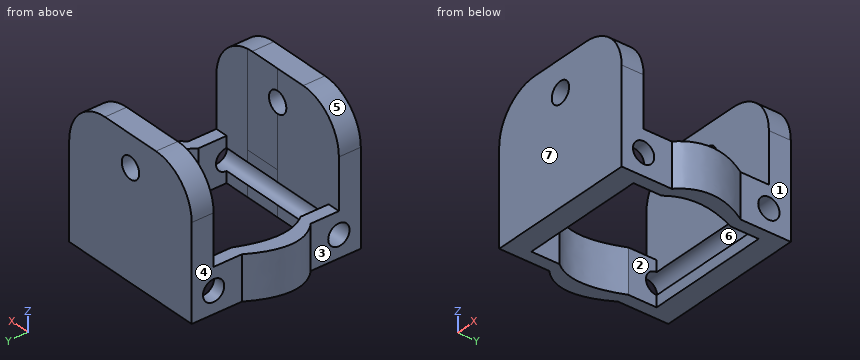
```python
from build123d import *

# Parameters (mm, degrees)
SKETCH1_W               = 24
SKETCH1_H               = 3.5
BOSS_EXTRUDE1_DEPTH     = 7
BOSS_EXTRUDE2_START     = 7
BOSS_EXTRUDE2_OUTLINE_W = 24
BOSS_EXTRUDE2_OUTLINE_H = 3.5
BOSS_EXTRUDE2_DEPTH     = 15
FILLET1_R               = 7
M3_CLEARANCE_HOLE1_D    = 3.4
M3_CLEARANCE_HOLE2_D    = 3.4


# Read off the part's stored shape, not the designer's step: Boss-Extrude2
with BuildPart() as part:
    # Sketch1 → Boss-Extrude1 (new body)
    with BuildSketch(Plane.XY):
        with Locations((0, 11.75)):
            Rectangle(SKETCH1_W, SKETCH1_H)
        with BuildLine():
            Line((-10, 10), (-12, 10))
            Line((-12, 10), (-12, 5.5))
            add(Edge.make_bspline(
                [(-12, 5.5), (-16.208168435, -1.452739177), (-12, -5.5)],
                knots=[0, 0, 0, 0.703674115, 0.703674115, 0.703674115], degree=2))
            Line((-12, -5.5), (-12, -10))
            Line((-12, -10), (-10, -10))
            Line((-10, -10), (-10, -5.5))
            add(Edge.make_bspline(
                [(-10, 5.5), (-13.144989471, -1.593519523), (-10, -5.5)],
                knots=[0, 0, 0, 0.703674115, 0.703674115, 0.703674115], degree=2))
            Line((-10, 5.5), (-10, 10))
        make_face()
        with BuildLine():
            Line((12, 5.5), (12, 10))
            Line((12, 10), (10, 10))
            Line((10, 10), (10, 5.5))
            add(Edge.make_bspline(
                [(10, 5.5), (13.144989471, -1.593519523), (10, -5.5)],
                knots=[0, 0, 0, 0.703674115, 0.703674115, 0.703674115], degree=2))
            Line((10, -5.5), (10, -10))
            Line((10, -10), (12, -10))
            Line((12, -10), (12, -5.5))
            add(Edge.make_bspline(
                [(12, 5.5), (16.208168435, -1.452739177), (12, -5.5)],
                knots=[0, 0, 0, 0.703674115, 0.703674115, 0.703674115], degree=2))
        make_face()
        with BuildLine():
            Line((-10, -10), (-12, -10))
            Line((-12, -10), (-12, -13.5))
            Line((-12, -13.5), (12, -13.5))
            Line((12, -13.5), (12, -10))
            Line((12, -10), (10, -10))
            Line((10, -10), (5.934098246, -10))
            add(Edge.make_bspline(
                [(5.934098246, -10), (5.478588927, -10.00932896), (0, -10)],
                knots=[0.968742805, 0.968742805, 0.968742805, 1, 1, 1], degree=2))
            Line((0, -10), (-10, -10))
        make_face()
    extrude(amount=BOSS_EXTRUDE1_DEPTH)

    # Boss-Extrude2 outline → Boss-Extrude2 (add)
    with BuildSketch(Plane.XY.offset(BOSS_EXTRUDE2_START)):
        with BuildLine():
            Line((12, -10), (5.934098246, -10))
            add(Edge.make_bspline(
                [(5.934098246, -10), (5.478588927, -10.00932896), (0, -10)],
                knots=[0.968742805, 0.968742805, 0.968742805, 1, 1, 1], degree=2))
            Line((0, -10), (-12, -10))
            Line((-12, -10), (-12, -13.5))
            Line((-12, -13.5), (12, -13.5))
            Line((12, -13.5), (12, -10))
        make_face()
        with Locations((0, 11.75)):
            Rectangle(BOSS_EXTRUDE2_OUTLINE_W, BOSS_EXTRUDE2_OUTLINE_H)
    extrude(amount=BOSS_EXTRUDE2_DEPTH)

    # Fillet1
    fillet1_edges = [part.edges().sort_by_distance(p)[0] for p in [
        (12, -11.75, 22),
        (-12, -11.75, 22),
        (12, 11.75, 22),
        (-12, 11.75, 22),
    ]]
    fillet(fillet1_edges, radius=FILLET1_R)

    # M3 Clearance Hole1 (through all)
    with Locations(Plane.ZY.offset(12)):
        with Locations((3.5, 10), (3.5, -10)):
            Hole(M3_CLEARANCE_HOLE1_D / 2)

    # M3 Clearance Hole2 (through all)
    with Locations(Plane(origin=(0, 13.5, 0), x_dir=(1, 0, 0), z_dir=(0, 1, 0))):
        with Locations((0, -17)):
            Hole(M3_CLEARANCE_HOLE2_D / 2)


solid = part.part
```
For this review, take the finished solid that the model builds, in its own axes (mm). Face numbers are marked on the shaded views. A direction names the side the tool comes from. Coordinates: 2 decimals unless noted, no trailing zeros. Loops run counter-clockwise (first coordinate to the right, second up) from the corner with the lowest first, then second, coordinate; pieces in that order, holes last. Notation, with made-up numbers: (34.25, 80.5) -> (66.25, 80.5) arc R17 ccw to (66.25, 109.5) -> close; hole circle Ø3 at (52.5, 59.25). An arc over 180 degrees is marked (long way). Return JSON: item names as keys, results as strings. Group by question number.
(1) To check wall thickness, follow L1, parallel to X at y = -11.8, z = 17; L2, parallel to Y at x = 7.5, z = 14; L3, parallel to Z at x = 0, y = 10.9. State the ranges of each line that lie inside material, in increasing order.
(2) Consider section B-B, the plane x = -4.5. Give the boundary of the cut face in (y, z).
(3) Tool access review of the marked faces 1, 2, 3 and 4: name each direction out of +Z, -Z, +X, -X, +Y, -Y from which nothing blocks a thin tool from reaching the whole face with its end or side.
(4) Consider section C-C, the plane z = 3.5. Count the separate pieces of the cut face and the enclosed holes in it, plus the area to 3 significant figures.
(5) Mouldability with a two-part tool opening along Z and no side actions: class the marked faces 5, 6 and 7 as pulls with the +Z half, pulls with the -Z half, needs draft (parallel to the pull), parting line crosses it, or undercut.
(6) Consider section D-D, the plane x = 7.5. Give the boundary of the cut face in (y, z).
(7) Consider section A-A, the plane y = -6.75. Give the boundary of the cut face in (x, z).
(8) For pin 1 Ø9 at (y, z) = (8.5, 4.5) entering from -X; pin 2 Ø10 at (x, y) = (-10, -7.5) entering from +Z; pin 3 Ø12 at (x, y) = (4.5, 2) entering from -Z; pin 4 Ø5 at (y, z) = (9, 3) entering from -X, all flat-tipped, find the tip position at first contact; note any pin that passes through.
Results below:
{
 "1": {"L1": "x = -11.71 to -1.7, 1.7 to 11.71", "L2": "y = -13.5 to -10, 10 to 13.5", "L3": "z = 0 to 2.06, 4.94 to 15.3, 18.7 to 22"},
 "2": {"outline": "(-13.5, 0) -> (-10, 0) -> (-10, 1.8) arc R1.7 cw to (-10, 5.2) -> (-10, 22) -> (-13.5, 22) -> close; (10, 0) -> (13.5, 0) -> (13.5, 22) -> (10, 22) -> (10, 5.2) arc R1.7 cw to (10, 1.8) -> close"},
 "3": {"face 1": "+Z, -Z, +X, +Y", "face 2": "+Z, -Z", "face 3": "+Z, -Z, -X, -Y", "face 4": "+Z, -Z, -X, +Y"},
 "4": {"separate pieces": "4", "enclosed holes": "0", "area": "161 mm2"},
 "5": {"face 5": "pulls with the +Z half", "face 6": "undercut", "face 7": "needs draft"},
 "6": {"outline": "(-13.5, 0) -> (-10, 0) -> (-10, 1.8) arc R1.7 cw to (-10, 5.2) -> (-10, 21.54) -> (-13.5, 21.54) -> close; (10, 0) -> (13.5, 0) -> (13.5, 21.54) -> (10, 21.54) -> (10, 5.2) arc R1.7 cw to (10, 1.8) -> close"},
 "7": {"outline": "(-12, 0) -> (-10, 0) -> (-10, 7) -> (-12, 7) -> close; (10, 0) -> (12, 0) -> (12, 7) -> (10, 7) -> close"},
 "8": {"pin 1": "stops at x = -12.83", "pin 2": "stops at z = 21.97", "pin 3": "passes through", "pin 4": "stops at x = -12"}
}
